Autodesk Inventor part; units mm, degrees
ref_plane "YZ Plane" through (0, 0, 0) normal (1, 0, 0) x (0, 1, 0)
ref_plane "XZ Plane" through (0, 0, 0) normal (0, 1, 0) x (-1, 0, 0)
ref_plane "XY Plane" through (0, 0, 0) normal (0, 0, 1) x (1, 0, 0)
sketch "Sketch1" plane through (0, 0, 0) normal (1, 0, 0) x (0, 1, 0)
  line L0 (-14.5623, 18.9434) -> (14.5623, 18.9434)
  line L1 (14.5623, 18.9434) -> (14.5623, -18.9434)
  line L2 (14.5623, -18.9434) -> (-14.5623, -18.9434)
  line L3 (-14.5623, -18.9434) -> (-14.5623, 18.9434)
  line L4 (-14.5623, 18.9434) -> (14.5623, -18.9434) construction
  line L5 (14.5623, 18.9434) -> (-14.5623, -18.9434) construction
  point P0 (0, 0)
extrude "Extrusion1" add sketch "Sketch1" along normal blind 60.3
sketch "Sketch2" plane through (60.3, 0, 0) normal (1, 0, 0) x (0, 0, -1)
  point P0 (0, 0)
  point P1 (1.6165, 1.4208)
hole "Hole1" at (60.3, 1.4208, -1.6165) direction (-1, 0, 0) diameter 14 end through all
properties part number "Pieza para tornillos"
Check sheet for the modelled part. Datum: model origin and axes. Units: mm. Give positions to 0.01 mm unless a question says otherwise; leave off trailing zeros. Write each loop counter-clockwise with the first axis right and the second up, starting at its lowest first coordinate (ties: lowest second). Pieces come first, ordered by that corner, then holes. Notation, with made-up numbers: (-12.5, 62.25) - (-4.5, 62.25) arc R10 ccw to (-4.5, 79.25) - close; hole circle Ø1 at (-25, 24.5). An arc over 180 degrees is marked (long way). Answer as a JSON object with one key per item and string values. Group by question number.
1) Thickness scan on probe 1 along Y at (x, z) = (11, -5); probe 2 along Z at (x, y) = (39.5, 0.5); probe 3 along Z at (x, y) = (15, 1). Record the ranges inside material, lowest first. Write a range as from..to.
2) Sectioned sample at A-A (y = 4). Record the cut outline in (x, z).
3) Sectioned sample at B-B (x = 49). Record the cut outline in (y, z).
4) Sectioned sample at C-C (y = -1). Record the cut outline in (x, z).
Geometry results:
{
 "1": {"probe 1": "y = -14.56..-4.71, 7.55..14.56", "probe 2": "z = -18.94..-8.56, 5.32..18.94", "probe 3": "z = -18.94..-8.6, 5.37..18.94"},
 "2": {"outline": "(0, -18.94) - (60.3, -18.94) - (60.3, -8.12) - (0, -8.12) - close; (0, 4.89) - (60.3, 4.89) - (60.3, 18.94) - (0, 18.94) - close"},
 "3": {"outline": "(-14.56, -18.94) - (14.56, -18.94) - (14.56, 18.94) - (-14.56, 18.94) - close; hole circle Ø14 at (1.42, -1.62)"},
 "4": {"outline": "(0, -18.94) - (60.3, -18.94) - (60.3, -8.18) - (0, -8.18) - close; (0, 4.95) - (60.3, 4.95) - (60.3, 18.94) - (0, 18.94) - close"}
}
